Here's how the part is built. I have some questions about the finished solid (model axes, mm). Face numbers are marked on the shaded views. A direction names the side the tool comes from. Round coordinates to 2 decimals unless told otherwise and drop trailing zeros. Order: outer loops, then holes, each group sorted by start corner. A loop starts at its lowest first (then second) coordinate and runs counter-clockwise, first axis right, second up. Notation, with made-up numbers: (-19.5, 46) - (38.5, 46) arc R32 cw to (38.5, 75) - close; hole circle Ø10 at (18.25, 70.25). An arc over 180 degrees is marked (long way). Answer as a JSON object with one key per item and string values.
```python
from build123d import *

# Parameters (mm, degrees)
SKETCH1_R               = 6.45
BOSS_EXTRUDE1_DEPTH     = 15
SKETCH2_W               = 5
SKETCH2_H               = 3
CUT_EXTRUDE3_DEPTH      = 5
CUT_EXTRUDE4_DEPTH      = 56.180796325
CUT_EXTRUDE4_DEPTH_BACK = 56.180796325
SKETCH4_R               = 1.5
SKETCH5_R               = 3
CUT_EXTRUDE5_DEPTH      = 4


with BuildPart() as part:
    # Sketch1 → Boss-Extrude1 (new body)
    with BuildSketch(Plane.XY):
        with BuildLine():
            Line((0, 23), (0, 37))
            Line((0, 37), (12.859510911, 37))
            Line((12.859510911, 37), (12.859510911, 27))
            ThreePointArc((12.859510911, 27), (20.383390121, 21.88342816), (26.020458433, 14.741192754))
            Line((26.020458433, 14.741192754), (28.050458433, 14.741192754))
            Line((28.050458433, 14.741192754), (28.050458433, 9.460443964))
            ThreePointArc((28.050458433, 9.460443964), (34.500458433, 11.45), (40.950458433, 9.460443964))
            Line((40.950458433, 9.460443964), (40.950458433, 35))
            Line((40.950458433, 35), (50.950458433, 35))
            Line((50.950458433, 35), (50.950458433, -35))
            Line((50.950458433, -35), (40.950458433, -35))
            Line((40.950458433, -35), (40.950458433, -9.460443964))
            ThreePointArc((40.950458433, -9.460443964), (34.500458433, -11.45), (28.050458433, -9.460443964))
            Line((28.050458433, -9.460443964), (28.050458433, -14.741192754))
            Line((28.050458433, -14.741192754), (26.020458433, -14.741192754))
            ThreePointArc((26.020458433, -14.741192754), (20.383390121, -21.88342816), (12.859510911, -27))
            Line((12.859510911, -27), (12.859510911, -37))
            Line((12.859510911, -37), (0, -37))
            Line((0, -37), (0, -23))
            ThreePointArc((0, -23), (23, 0), (0, 23))
        make_face()
        with Locations(Location((34.500458433, 0, 0), (0, 0, 180))):
            Circle(SKETCH1_R, mode=Mode.SUBTRACT)
    extrude(amount=BOSS_EXTRUDE1_DEPTH)

    # Sketch2 → Cut-Revolve1 (revolve, cut)
    with BuildSketch(Plane.ZY):
        with Locations((7.5, 24.5)):
            Rectangle(SKETCH2_W, SKETCH2_H)
    revolve(axis=Axis((0, 0, 15), (0, 0, -1)), mode=Mode.SUBTRACT)

    # Sketch3 → Cut-Extrude3 (cut)
    with BuildSketch(Plane(origin=(50.950458433, 0, 0), x_dir=(0, 0, -1), z_dir=(1, 0, 0))):
        with BuildLine():
            Line((-12.5, -25), (-12.5, 25))
            ThreePointArc((-12.5, 25), (-7.5, 30), (-2.5, 25))
            Line((-2.5, 25), (-2.5, -25))
            ThreePointArc((-2.5, -25), (-7.5, -30), (-12.5, -25))
        make_face()
    extrude(amount=-CUT_EXTRUDE3_DEPTH, mode=Mode.SUBTRACT)

    # Sketch4 → Cut-Extrude4 (cut, two sides: drawn at the far end of the back side and taken through both)
    with BuildSketch(Plane(origin=(12.859510911, 0, 0), x_dir=(0, 0, -1), z_dir=(1, 0, 0)).offset(-CUT_EXTRUDE4_DEPTH_BACK)):
        with Locations((-7.333431897, 32)):
            Circle(SKETCH4_R)
        with Locations((-7.333431897, -32)):
            Circle(SKETCH4_R)
    extrude(amount=CUT_EXTRUDE4_DEPTH + CUT_EXTRUDE4_DEPTH_BACK, mode=Mode.SUBTRACT)

    # Sketch5 → Cut-Extrude5 (cut)
    with BuildSketch(Plane(origin=(12.859510911, 0, 0), x_dir=(0, 0, -1), z_dir=(1, 0, 0))):
        with Locations((-7.5, 32)):
            Circle(SKETCH5_R)
        with Locations(Location((-7.5, -32, 0), (0, 0, 180))):
            Circle(SKETCH5_R)
    extrude(amount=-CUT_EXTRUDE5_DEPTH, mode=Mode.SUBTRACT)


solid = part.part
```
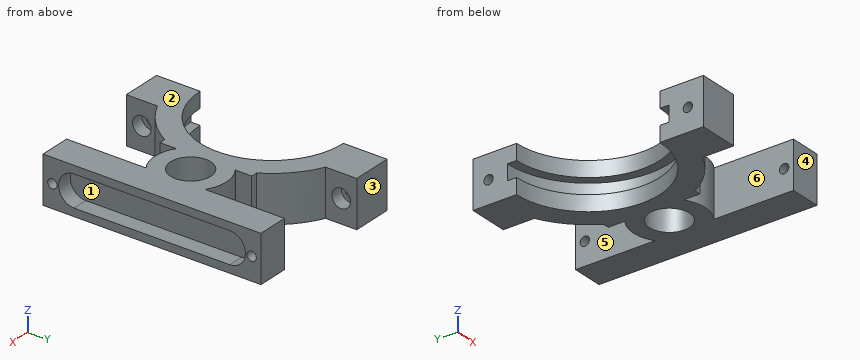
1. Imagine slicing it at B-B (x = 7). List the corners of the cut face in (y, z) for me.
Responses:
{"outline": "(-37, 0) - (-21.91, 0) - (-21.91, 5) - (-25.04, 5) - (-25.04, 10) - (-21.91, 10) - (-21.91, 15) - (-37, 15) - close; (21.91, 0) - (37, 0) - (37, 15) - (21.91, 15) - (21.91, 10) - (25.04, 10) - (25.04, 5) - (21.91, 5) - close; hole circle Ø3 at (-32, 7.33); hole circle Ø3 at (32, 7.33)"}
2. Thinking about a two-plate mould opening in Y: for the marked faces 1, 2 and 3, which applies, pulls with the +Y half, pulls with the -Y half, needs draft (parallel to the pull), parting line crosses it, or undercut?
Responses:
{"face 1": "undercut", "face 2": "needs draft", "face 3": "pulls with the +Y half"}
3. For the marked faces 4, 5 and 6, which set-ups out of +Z, -Z, +X, -X, +Y, -Y let a thin tool reach every point of the face, with its end or its side?
Responses:
{"face 4": "+Z, -Z, +X, -Y", "face 5": "+Z, -Z, +Y", "face 6": "+Z, -Z, -Y"}
4. If I drill on L1, parallel to Z at x = 22.5, y = -6.5; L2, parallel to Z at x = 47, y = -32; L3, parallel to Y at x = 10.65, z = 7.5, over which ranges is the centre line in solid material (lowest first)? Write a range as [from, to].
Responses:
{"L1": "[0, 5], [10, 15]", "L2": "[0, 5.83], [8.83, 15]", "L3": "[-37, -35], [-29, -23.72], [23.72, 29], [35, 37]"}
5. For P1, Ø7.5, axis at x = 34.5, y = 0, coming from the -Z side; P2, Ø8, axis at y = -16.5, z = 7.5, coming from the -X side; P3, Ø3, axis at y = -7, z = 9, coming from the -X side, each with a flat end and sliding along its axis, tell me the tip position at first contact or that it passes through.
Responses:
{"P1": "through", "P2": "x = 12", "P3": "x = 21.52"}
6. Imagine slicing it at A-A (y = 32). List the corners of the cut face in (x, z) for me, plus the area to 3 significant figures.
Responses:
{"outline": "(0, 0) - (12.86, 0) - (12.86, 4.5) - (8.86, 4.5) - (8.86, 5.83) - (0, 5.83) - close; (0, 8.83) - (8.86, 8.83) - (8.86, 10.5) - (12.86, 10.5) - (12.86, 15) - (0, 15) - close; (40.95, 0) - (50.95, 0) - (50.95, 5.83) - (40.95, 5.83) - close; (40.95, 8.83) - (50.95, 8.83) - (50.95, 15) - (40.95, 15) - close", "area": "262 mm2"}
7. Imagine slicing it at C-C (y = 4.5). List the corners of the cut face in (x, z) for me.
Responses:
{"outline": "(22.56, 0) - (29.88, 0) - (29.88, 15) - (22.56, 15) - (22.56, 10) - (25.61, 10) - (25.61, 5) - (22.56, 5) - close; (39.12, 0) - (50.95, 0) - (50.95, 2.5) - (45.95, 2.5) - (45.95, 12.5) - (50.95, 12.5) - (50.95, 15) - (39.12, 15) - close"}
8. Imagine slicing it at D-D (x = 20.5). List the corners of the cut face in (y, z) for me, plus the area to 3 significant figures.
Responses:
{"outline": "(-21.77, 0) - (-10.43, 0) - (-10.43, 5) - (-15.99, 5) - (-15.99, 10) - (-10.43, 10) - (-10.43, 15) - (-21.77, 15) - close; (10.43, 0) - (21.77, 0) - (21.77, 15) - (10.43, 15) - (10.43, 10) - (15.99, 10) - (15.99, 5) - (10.43, 5) - close", "area": "285 mm2"}
